For this review, take the finished solid that the model builds, in its own axes (mm). A direction names the side the tool comes from. Round coordinates to 2 decimals unless told otherwise and drop trailing zeros. Write each loop counter-clockwise with the first axis right and the second up, starting at its lowest first coordinate (ties: lowest second). Pieces come first, ordered by that corner, then holes.
from build123d import *

# Parameters (mm, degrees)
MODEL_R                 = 1.5
SALIENTE_EXTRUIR1_DEPTH = 3


with BuildPart() as part:
    # Model → Saliente-Extruir1 (new body)
    with BuildSketch(Plane.XY):
        with BuildLine():
            Line((183.097853309, 273.646547335), (201.097853309, 273.646547335))
            ThreePointArc((201.097853309, 273.646547335), (205.597853309, 269.146547335), (201.097853309, 264.646547335))
            Line((201.097853309, 264.646547335), (183.097853309, 264.646547335))
            Line((183.097853309, 264.646547335), (183.097853309, 273.646547335))
        make_face()
        with Locations((201.097853309, 269.146547335)):
            Circle(MODEL_R, mode=Mode.SUBTRACT)
        with BuildLine():
            Line((186.722853309, 265.896547335), (188.472853309, 265.896547335))
            ThreePointArc((188.472853309, 265.896547335), (189.003183395, 266.116217249), (189.222853309, 266.646547335))
            Line((189.222853309, 266.646547335), (189.222853309, 271.646547335))
            ThreePointArc((189.222853309, 271.646547335), (189.003183395, 272.176877421), (188.472853309, 272.396547335))
            Line((188.472853309, 272.396547335), (186.722853309, 272.396547335))
            ThreePointArc((186.722853309, 272.396547335), (186.192523223, 272.176877421), (185.972853309, 271.646547335))
            Line((185.972853309, 271.646547335), (185.972853309, 266.646547335))
            ThreePointArc((185.972853309, 266.646547335), (186.192523223, 266.116217249), (186.722853309, 265.896547335))
        make_face(mode=Mode.SUBTRACT)
    extrude(amount=SALIENTE_EXTRUIR1_DEPTH)


solid = part.part
(1) For faces 1 (the face through (185.973, 269, 1)), 2 (the face through (195, 269, 3)), list the 3-axis set-ups (+Z, -Z, +X, -X, +Y, -Y) from which the entire face can be reached by the end or side of a thin tool; tool diameter is ignored.
Geometry check:
face 1: +Z, -Z
face 2: +Z, +X, -X, +Y, -Y
(2) Mouldability with a two-part tool opening along Y and no side actions: class faces 3 (the face through (192, 273.647, 1)), 4 (the face through (188, 272.397, 1)), 5 (the face through (205.597, 269.245, 1.479)) as pulls with the +Y half, pulls with the -Y half, needs draft (parallel to the pull), parting line crosses it, or undercut.
Geometry check:
face 3: pulls with the +Y half
face 4: undercut
face 5: parting line crosses it
(3) We need section B-B, the plane y = 270. Give the boundary of the cut face in (x, z).
Geometry check:
outline: (183.1, 0) - (185.97, 0) - (185.97, 3) - (183.1, 3) - close; (189.22, 0) - (199.86, 0) - (199.86, 3) - (189.22, 3) - close; (202.33, 0) - (205.52, 0) - (205.52, 3) - (202.33, 3) - close
(4) For line 1 along Y through (x, z) = (187, 1); line 2 along X through (y, z) = (268.5, 2.15); line 3 along X through (y, z) = (269.5, 0.7), list the stretches that pass through material, from the lowest coordinate up.
Geometry check:
line 1: y = 264.65 to 265.9, 272.4 to 273.65
line 2: x = 183.1 to 185.97, 189.22 to 199.74, 202.45 to 205.55
line 3: x = 183.1 to 185.97, 189.22 to 199.64, 202.56 to 205.58
(5) We need section C-C, the plane y = 272. Give the boundary of the cut face in (x, z).
Geometry check:
outline: (183.1, 0) - (186.06, 0) - (186.06, 3) - (183.1, 3) - close; (189.13, 0) - (204.58, 0) - (204.58, 3) - (189.13, 3) - close
(6) We need section A-A, the plane x = 188. Give the boundary of the cut face in (y, z), and give its area (3 significant figures).
Geometry check:
outline: (264.65, 0) - (265.9, 0) - (265.9, 3) - (264.65, 3) - close; (272.4, 0) - (273.65, 0) - (273.65, 3) - (272.4, 3) - close
area: 7.50 mm2
(7) We need section D-D, the plane z = 0.7. Give the boundary of the cut face in (x, y).
Geometry check:
outline: (183.1, 264.65) - (201.1, 264.65) arc R4.5 ccw to (201.1, 273.65) - (183.1, 273.65) - close; hole (185.97, 266.65) arc R0.75 ccw to (186.72, 265.9) - (188.47, 265.9) arc R0.75 ccw to (189.22, 266.65) - (189.22, 271.65) arc R0.75 ccw to (188.47, 272.4) - (186.72, 272.4) arc R0.75 ccw to (185.97, 271.65) - close; hole circle Ø3 at (201.1, 269.15)
